For this review, take the finished solid that the model builds, in its own axes (mm). Face numbers are marked on the shaded views. A direction names the side the tool comes from. Give positions to 0.01 mm unless a question says otherwise; leave off trailing zeros. Loops run counter-clockwise (first coordinate to the right, second up) from the corner with the lowest first, then second, coordinate; pieces in that order, holes last. Notation, with made-up numbers: (43, -30) - (90, -30) arc R21 cw to (90, -13) - close; hole circle Ø7 at (8, 73). An arc over 180 degrees is marked (long way). Use CSV: the item, a comma, the result in double quotes. Start each with the question number.
1. Take a section at D-D on x = 3. Give the boundary of the cut face in (y, z), plus the area to 3 significant figures.
2. Wall thickness on line 1 (Y direction, x = -8, z = 27.7); line 2 (Z direction, x = 1.5, y = -6.75); line 3 (Z direction, x = -9.75, y = 7.5): over which ranges is each line inside the solid? List them lowest first.
3. Take a section at A-A on z = 27.5. Give the boundary of the cut face in (x, y).
4. For pin 1 (2 mm diameter, centred on x = -4.5, y = -3.5, fed in from +Z); pin 2 (1.4 mm diameter, centred on x = 8, y = -8, fed in from +Z); pin 3 (2 mm diameter, centred on x = -11.5, z = 6, fed in from +Y), all flat-tipped, find the tip position at first contact; note any pin that passes through.
5. Take a section at B-B on z = 18.5. Give the boundary of the cut face in (x, y), plus the area to 3 significant figures.
6. For the marked faces 1 and 2, list the 3-axis set-ups (+Z, -Z, +X, -X, +Y, -Y) from which the entire face can be reached by the end or side of a thin tool; tool diameter is ignored.
7. Take a section at C-C on y = 0. Give the boundary of the cut face in (x, z), plus the area to 3 significant figures.
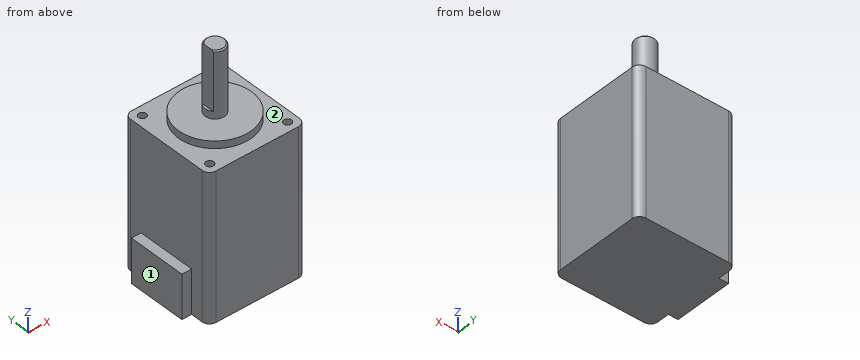
```python
from build123d import *

# Parameters (mm, degrees)
SKETCH004_W     = 20
SKETCH004_H     = 20
PAD003_DEPTH    = 30
SKETCH005_R     = 7.5
PAD004_DEPTH    = 1.5
FILLET_R        = 1.5
SKETCH006_R     = 0.8
HOLE_DEPTH      = 3.019312
HOLE_TIPS_R     = 0.8
SKETCH007_R     = 2
PAD005_DEPTH    = 13.5
SKETCH008_W     = 5
SKETCH008_H     = 10
POCKET001_DEPTH = 12
CHAMFER001_SIZE = 0.25
SKETCH009_W     = 12
SKETCH009_H     = 9
PAD006_DEPTH    = 2


with BuildPart() as part:
    # Sketch004 → Pad003 (new body)
    with BuildSketch(Plane.XY):
        Rectangle(SKETCH004_W, SKETCH004_H)
    extrude(amount=PAD003_DEPTH)

    # Sketch005 (on Face6 of Pad003) → Pad004 (join)
    with BuildSketch(Plane.XY.offset(30)):
        Circle(SKETCH005_R)
    extrude(amount=PAD004_DEPTH)

    # Fillet
    fillet_edges = [part.edges().sort_by_distance(p)[0] for p in [
        (-10, -10, 15),
        (10, -10, 15),
        (10, 10, 15),
        (-10, 10, 15),
    ]]
    fillet(fillet_edges, radius=FILLET_R)

    # Sketch006 (on Face5 of Fillet) → Hole (cut)
    with BuildSketch(Plane.XY.offset(30)):
        with Locations((-8, 8)):
            Circle(SKETCH006_R)
        with Locations((8, 8)):
            Circle(SKETCH006_R)
        with Locations((8, -8)):
            Circle(SKETCH006_R)
        with Locations((-8, -8)):
            Circle(SKETCH006_R)
    extrude(amount=-HOLE_DEPTH, mode=Mode.SUBTRACT)

    # Hole tips → Hole tip 1 section 0
    with BuildSketch(Plane.XY.offset(26.980688), mode=Mode.PRIVATE) as hole_tip_1_s0:
        with Locations((-8, 8)):
            Circle(HOLE_TIPS_R)
    loft([hole_tip_1_s0.sketch, Vertex(-8, 8, 26.5)], mode=Mode.SUBTRACT)

    # Hole tips → Hole tip 2 section 0
    with BuildSketch(Plane.XY.offset(26.980688), mode=Mode.PRIVATE) as hole_tip_2_s0:
        with Locations((8, 8)):
            Circle(HOLE_TIPS_R)
    loft([hole_tip_2_s0.sketch, Vertex(8, 8, 26.5)], mode=Mode.SUBTRACT)

    # Hole tips → Hole tip 3 section 0
    with BuildSketch(Plane.XY.offset(26.980688), mode=Mode.PRIVATE) as hole_tip_3_s0:
        with Locations((8, -8)):
            Circle(HOLE_TIPS_R)
    loft([hole_tip_3_s0.sketch, Vertex(8, -8, 26.5)], mode=Mode.SUBTRACT)

    # Hole tips → Hole tip 4 section 0
    with BuildSketch(Plane.XY.offset(26.980688), mode=Mode.PRIVATE) as hole_tip_4_s0:
        with Locations((-8, -8)):
            Circle(HOLE_TIPS_R)
    loft([hole_tip_4_s0.sketch, Vertex(-8, -8, 26.5)], mode=Mode.SUBTRACT)

    # Sketch007 (on Face17 of Hole) → Pad005 (join)
    with BuildSketch(Plane.XY.offset(31.5)):
        Circle(SKETCH007_R)
    extrude(amount=PAD005_DEPTH)

    # Sketch008 (on Face22 of Pad005) → Pocket001 (cut)
    with BuildSketch(Plane.XY.offset(45)):
        with Locations((-4, 0)):
            Rectangle(SKETCH008_W, SKETCH008_H)
    extrude(amount=-POCKET001_DEPTH, mode=Mode.SUBTRACT)

    # Chamfer001
    chamfer001_edges = [part.edges().sort_by_distance(p)[0] for p in [
        (0.707107, -1.870829, 45),
        (0.707107, 1.870829, 45),
    ]]
    chamfer(chamfer001_edges, length=CHAMFER001_SIZE)

    # Sketch009 (on Face13 of Chamfer001) → Pad006 (join)
    with BuildSketch(Plane(origin=(-10, 0, 0), x_dir=(0, -1, 0), z_dir=(-1, 0, 0))):
        with Locations((0, 4.5)):
            Rectangle(SKETCH009_W, SKETCH009_H)
    extrude(amount=PAD006_DEPTH)


solid = part.part
```
Check result:
1,outline,"(-10, 0) - (10, 0) - (10, 30) - (6.87, 30) - (6.87, 31.5) - (-6.87, 31.5) - (-6.87, 30) - (-10, 30) - close"
1,area,"621 mm²"
2,line 1,"y = -10 to -8.8, -7.2 to 7.2, 8.8 to 10"
2,line 2,"z = 0 to 31.5"
2,line 3,"z = 0 to 30"
3,outline,"(-10, -8.5) arc R1.5 ccw to (-8.5, -10) - (8.5, -10) arc R1.5 ccw to (10, -8.5) - (10, 8.5) arc R1.5 ccw to (8.5, 10) - (-8.5, 10) arc R1.5 ccw to (-10, 8.5) - close; hole circle Ø1.6 at (-8, -8); hole circle Ø1.6 at (-8, 8); hole circle Ø1.6 at (8, -8); hole circle Ø1.6 at (8, 8)"
4,pin 1,"stops at z = 31.5"
4,pin 2,"stops at z = 26.92"
4,pin 3,"stops at y = 6"
5,outline,"(-10, -8.5) arc R1.5 ccw to (-8.5, -10) - (8.5, -10) arc R1.5 ccw to (10, -8.5) - (10, 8.5) arc R1.5 ccw to (8.5, 10) - (-8.5, 10) arc R1.5 ccw to (-10, 8.5) - close"
5,area,"398 mm²"
6,face 1,"+Z, -Z, -X, +Y, -Y"
6,face 2,"+Z"
7,outline,"(-12, 0) - (10, 0) - (10, 30) - (7.5, 30) - (7.5, 31.5) - (2, 31.5) - (2, 44.75) - (1.75, 45) - (-1.5, 45) - (-1.5, 33) - (-2, 33) - (-2, 31.5) - (-7.5, 31.5) - (-7.5, 30) - (-10, 30) - (-10, 9) - (-12, 9) - close"
7,area,"688 mm²"
